```python
from build123d import *

# Parameters (mm, degrees)
PAD014_DEPTH    = 243
SKETCH010_R     = 4.925
POCKET_DEPTH    = 20
SKETCH013_W     = 3
SKETCH013_H     = 207
POCKET001_DEPTH = 5


with BuildPart() as part:
    # Sketch009 → Pad014 (new body)
    with BuildSketch(Plane.XY):
        Polygon((0, 206.4), (0, 196.4), (13, 196.4), (13, 182.4), (0, 182.4), (0, 157), (13, 157), (13, 116.4), (0, 116.4), (0, 91), (13, 91), (13, 50.4), (0, 50.4), (0, 25), (13, 25), (13, 10), (0, 10), (0, 0), (23, 0), (23, 206.4), align=None)
    extrude(amount=PAD014_DEPTH)

    # Sketch010 (on Vertex37 of Pad014) → Pocket (cut)
    with BuildSketch(Plane(origin=(23, 0, 0), x_dir=(-1, 0, 0), z_dir=(0, 0, -1))):
        with Locations((14, 104)):
            Circle(SKETCH010_R)
        with Locations((14, 170)):
            Circle(SKETCH010_R)
        with Locations((14, 38)):
            Circle(SKETCH010_R)
    extrude(amount=-POCKET_DEPTH, mode=Mode.SUBTRACT)

    # Sketch013 (on Face6 of Pocket) → Pocket001 (cut)
    with BuildSketch(Plane(origin=(23, 0, 0), x_dir=(0, 0, -1), z_dir=(1, 0, 0))):
        with Locations((-1.5, 103.5)):
            Rectangle(SKETCH013_W, SKETCH013_H)
    extrude(amount=-POCKET001_DEPTH, mode=Mode.SUBTRACT)

    # Mirrored: part across face of Pocket


with BuildPart() as part_1:
    add(part.part)
    add(part.part.mirror(Plane(origin=(13.661045, 103.34943, 243), x_dir=(1, 0, 0), z_dir=(0, 0, 1))))


with BuildPart() as part_2:
    # Body010 placement: moved
    add(part_1.part.moved(Location((440.6, 14.75, 284))))


solid = part_2.part
```
Could you check a few things on this model? Use its own coordinates, in mm. A direction names the side the tool comes from. Give positions to 0.01 mm unless a question says otherwise; leave off trailing zeros. Loops run counter-clockwise (first coordinate to the right, second up) from the corner with the lowest first, then second, coordinate; pieces in that order, holes last. Notation, with made-up numbers: (87, -37) - (146, -37) arc R5 cw to (146, -32) - close; hole circle Ø7 at (64, 56.5). An arc over 180 degrees is marked (long way). Answer in a Markdown table with one row per item. Add a question column.
Q1. Please list where these lines run through material, in increasing order: L1, parallel to Y at x = 445.5, z = 348.5; L2, parallel to X at y = 184, z = 756; L3, parallel to X at y = 171, z = 600.5. Write a range as from..to.
Q2. Which directions (+Z, -Z, +X, -X, +Y, -Y) give clear straight access to the entire face, cutting with the end or side of a thin tool? Please do faces 1 (the face through (447, 211.15, 530)), 2 (the face through (450, 185, 304)), 3 (the face through (454.52, 118.97, 760.14)).
Q3. If we section it at A-A (y = 52.75): List the corners of the cut face in (x, z) for me (3 decimals).
Q4. If we section it at C-C (x = 449.6): State how many separate pieces and enclosed holes the cut face has, plus the area to 3 significant figures.
Q5. We'd pull the mould along Y, two halves only. Please class faces 4 (the face through (440.6, 53, 530)), 5 (the face through (452, 221.15, 530)), 6 (the face through (453.6, 204, 530)): +Y half, -Y half, draft (parallel to the pull), parting line (faces both ways), or undercut.
Q6. For pin 1 (0.9 mm diameter, centred on y = 165.5, z = 768, fed in from +X); pin 2 (4 mm diameter, centred on x = 461.5, y = 57.5, fed in from -Z); pin 3 (9 mm diameter, centred on x = 449.6, y = 52.75, fed in from -Z); pin 4 (1 mm diameter, centred on x = 452.5, y = 78.5, fed in from +Z), each with a flat end and sliding along its axis, tell me the tip position at first contact or that it passes through.
Q7. If we section it at B-B (z = 663.5): List the corners of the cut face in (x, y) for me.
The answers:
| question | item | result |
|---|---|---|
| 1 | L1 | y = 14.75..24.75, 39.75..65.15, 105.75..131.15, 171.75..197.15, 211.15..221.15 |
| 1 | L2 | x = 440.6..444.73, 454.47..463.6 |
| 1 | L3 | x = 453.6..463.6 |
| 2 | face 1 | +Z, -Z, -X |
| 2 | face 2 | -Z |
| 2 | face 3 | +Z |
| 3 | outline | (440.6, 284) - (444.675, 284) - (444.675, 304) - (454.525, 304) - (454.525, 284) - (458.6, 284) - (458.6, 287) - (463.6, 287) - (463.6, 767) - (458.6, 767) - (458.6, 770) - (454.525, 770) - (454.525, 750) - (444.675, 750) - (444.675, 770) - (440.6, 770) - close |
| 4 | separate pieces | 5 |
| 4 | enclosed holes | 0 |
| 4 | area | 45,600 mm^2 |
| 5 | face 4 | draft |
| 5 | face 5 | +Y half |
| 5 | face 6 | undercut |
| 6 | pin 1 | stops at x = 458.6 |
| 6 | pin 2 | stops at z = 287 |
| 6 | pin 3 | stops at z = 304 |
| 6 | pin 4 | passes through |
| 7 | outline | (440.6, 14.75) - (463.6, 14.75) - (463.6, 221.15) - (440.6, 221.15) - (440.6, 211.15) - (453.6, 211.15) - (453.6, 197.15) - (440.6, 197.15) - (440.6, 171.75) - (453.6, 171.75) - (453.6, 131.15) - (440.6, 131.15) - (440.6, 105.75) - (453.6, 105.75) - (453.6, 65.15) - (440.6, 65.15) - (440.6, 39.75) - (453.6, 39.75) - (453.6, 24.75) - (440.6, 24.75) - close |
